Source: CAD feature listing. Evaluate the final solid. Frame: model axes, mm. Coordinates: 2 decimals unless noted, no trailing zeros. Write each loop counter-clockwise with the first axis right and the second up, starting at its lowest first coordinate (ties: lowest second). Pieces come first, ordered by that corner, then holes. Notation, with made-up numbers: M 37,19.25 L 82,19.25 A22 cw 82,42.25 Z; hole C 67,80 d2. An arc over 180 degrees is marked long. One line per item, written item: value. Start each with the question number.
Item 1: Ray query, L1, parallel to X at y = 8.5, z = 1; L2, parallel to X at y = 5.5, z = 3; L3, parallel to Y at x = 135.5, z = 6.5. Return the intervals inside material, ascending. Write a range as from..to.
Item 2: Cut plane A-A, the plane z = 3.5. Output: boundary loops of the cut face in (x, y).
Item 3: Cut plane C-C, the plane y = -11. Output: boundary loops of the cut face in (x, z).
Item 4: Mould query, pull axis X, two halves, no side actions, for faces 1 (the flat face through (165, 0, 4)), 2 (the cylindrical face through (-152.94, -8.77, 4.06)), 3 (the flat face through (-165, 0, 4)). Classes: released by +X, released by -X, zero draft, split by the parting line, or undercut.
Item 5: Cut plane B-B, the plane x = 0. Output: boundary loops of the cut face in (y, z).
```python
from build123d import *

# Parameters (mm, degrees)
SKETCH2_W           = 330
SKETCH2_H           = 38
BOSS_EXTRUDE1_DEPTH = 8
SKETCH3_R           = 7
CUT_EXTRUDE1_DEPTH  = 9
SKETCH4_R           = 3.3
CUT_EXTRUDE2_DEPTH  = 9


with BuildPart() as part:
    # Sketch2 → Boss-Extrude1 (new body)
    with BuildSketch(Plane.XY):
        Rectangle(SKETCH2_W, SKETCH2_H)
    extrude(amount=BOSS_EXTRUDE1_DEPTH)

    # Sketch3 → Cut-Extrude1 (cut, through all)
    with BuildSketch(Plane.XY.offset(8)):
        Circle(SKETCH3_R)
    extrude(amount=-CUT_EXTRUDE1_DEPTH, mode=Mode.SUBTRACT)

    # Sketch4 → Cut-Extrude2 (cut, through all)
    with BuildSketch(Plane.XY.offset(8)):
        with Locations((-135.508311731, 7)):
            Circle(SKETCH4_R)
        with Locations((-120.508311731, -11)):
            Circle(SKETCH4_R)
        with Locations((-150.508311731, -11)):
            Circle(SKETCH4_R)
    cut_extrude2 = extrude(amount=-CUT_EXTRUDE2_DEPTH, mode=Mode.SUBTRACT)

    # Mirror1: Cut-Extrude2 across plane
    add(cut_extrude2.mirror(Plane(origin=(0, 0, 0), x_dir=(0, 0, 1), z_dir=(1, 0, 0))), mode=Mode.SUBTRACT)


solid = part.part
```
From the geometry:
1. L1: x = -165..-138.45, -132.57..132.57, 138.45..165
1. L2: x = -165..-138.45, -132.57..-4.33, 4.33..132.57, 138.45..165
1. L3: y = -19..3.7, 10.3..19
2. outline: M -165,-19 L 165,-19 L 165,19 L -165,19 Z; hole C -150.51,-11 d6.6; hole C -135.51,7 d6.6; hole C -120.51,-11 d6.6; hole C 0,0 d14; hole C 120.51,-11 d6.6; hole C 135.51,7 d6.6; hole C 150.51,-11 d6.6
3. outline: M -165,0 L -153.81,0 L -153.81,8 L -165,8 Z; M -147.21,0 L -123.81,0 L -123.81,8 L -147.21,8 Z; M -117.21,0 L 117.21,0 L 117.21,8 L -117.21,8 Z; M 123.81,0 L 147.21,0 L 147.21,8 L 123.81,8 Z; M 153.81,0 L 165,0 L 165,8 L 153.81,8 Z
4. face 1: released by +X
4. face 2: undercut
4. face 3: released by -X
5. outline: M -19,0 L -7,0 L -7,8 L -19,8 Z; M 7,0 L 19,0 L 19,8 L 7,8 Z
